Design review of the part built by this model. Coordinates are the model's own, in mm. A direction names the side the tool comes from. Coordinates: 2 decimals unless noted, no trailing zeros. Write each loop counter-clockwise with the first axis right and the second up, starting at its lowest first coordinate (ties: lowest second). Pieces come first, ordered by that corner, then holes. Notation, with made-up numbers: (-7, 17.5) -> (35, 17.5) arc R21 cw to (35, 28.5) -> close; hole circle Ø11 at (53.5, 52). An arc over 180 degrees is marked (long way). Return JSON: item names as keys, results as strings. Group by question number.
from build123d import *

# Parameters (mm, degrees)
BOSS_EXTRUDE1_DEPTH = 9
CUT_EXTRUDE1_DEPTH  = 52
SKETCH4_W           = 7.545775994
SKETCH4_H           = 9.202794467
SKETCH4_W_2         = 8.134906164
CUT_EXTRUDE2_DEPTH  = 25


with BuildPart() as part:
    # Sketch2 → Boss-Extrude1 (new body)
    with BuildSketch(Plane.XY):
        with BuildLine():
            Line((-10.152941176, 19.036764706), (-10.152941176, 26.411764706))
            Line((-10.152941176, 26.411764706), (-38.352941176, 26.411764706))
            Line((-38.352941176, 26.411764706), (-38.352941176, -24.588235294))
            Line((-38.352941176, -24.588235294), (27.647058824, -24.588235294))
            Line((27.647058824, -24.588235294), (27.647058824, 26.411764706))
            Line((27.647058824, 26.411764706), (-0.552941176, 26.411764706))
            Line((-0.552941176, 26.411764706), (-0.552941176, 19.036764706))
            ThreePointArc((-0.552941176, 19.036764706), (-5.352941176, 14.236764706), (-10.152941176, 19.036764706))
        make_face()
    extrude(amount=BOSS_EXTRUDE1_DEPTH)

    # Sketch3 → Cut-Extrude1 (cut, through all)
    with BuildSketch(Plane(origin=(0, 26.411764706, 0), x_dir=(1, 0, 0), z_dir=(0, 1, 0))):
        Polygon((28.053319282, 0), (20.402615126, -2.05), (20.402615126, 0), align=None)
        Polygon((28.053319282, -9), (20.402615126, -6.95), (20.402615126, -9), align=None)
        Polygon((-38.759201635, 0), (-31.108497479, -2.05), (-31.108497479, 0), align=None)
        Polygon((-38.759201635, -9), (-31.108497479, -6.95), (-31.108497479, -9), align=None)
    extrude(amount=-CUT_EXTRUDE1_DEPTH, mode=Mode.SUBTRACT)

    # Sketch4 → Cut-Extrude2 (cut)
    with BuildSketch(Plane.XZ.offset(24.588235294)):
        with Locations((-34.881385476, 4.601397234)):
            Rectangle(SKETCH4_W, SKETCH4_H)
        with Locations((24.470068208, 4.601397234)):
            Rectangle(SKETCH4_W_2, SKETCH4_H)
    extrude(amount=-CUT_EXTRUDE2_DEPTH, mode=Mode.SUBTRACT)


solid = part.part
Q1. We need section A-A on y = 20.5. Write out the cut boundary in (x, z), plus the area to 3 significant figures.
Q2. We need section D-D on y = 3.5. Write out the cut boundary in (x, z).
Q3. For faces 5 (the flat face through (-34.781, 13.594, 7.934)), 6 (the flat face through (-34.781, 13.594, 1.066)), 7 (the flat face through (20.403, -4, 5)), list the 3-axis set-ups (+Z, -Z, +X, -X, +Y, -Y) from which the entire face can be reached by the end or side of a thin tool; tool diameter is ignored.
Q4. We need section C-C on z = 4.25. Write out the cut boundary in (x, y).
Q5. The part is to be moulded in two halves that separate along X. For faces 1 (the flat face through (14, 26.412, 4)), 2 (the flat face through (27.647, 13, 4)), 3 (the flat face through (-31.108, -4, 5)), 4 (the flat face through (-38.353, 14, 4)), say which applies: +X half, -X half, draft (parallel to the pull), parting line (faces both ways), or undercut.
Q6. We need section B-B on z = 1. Write out the cut boundary in (x, y).
Q7. For P1, Ø3.5, axis at x = 23, z = 5, coming from the -Y side; P2, Ø2.5, axis at y = -10, z = 4.5, coming from the -X side; P3, Ø1.5, axis at y = -14.5, z = 3, coming from the +X side, all flat-tipped, find the tip position at first contact; note any pin that passes through.
Q8. Wall thickness on L1, parallel to X at y = 20, z = 6.5; L2, parallel to X at y = -10.5, z = 4; L3, parallel to Y at x = 21, z = 6: over which ranges is each line inside the solid? List them lowest first.
Findings below:
{
 "1": {"outline": "(-38.35, 0.11) -> (-31.11, 2.05) -> (-31.11, 0) -> (-10.15, 0) -> (-10.15, 9) -> (-31.11, 9) -> (-31.11, 6.95) -> (-38.35, 8.89) -> close; (-0.55, 0) -> (20.4, 0) -> (20.4, 2.05) -> (27.65, 0.11) -> (27.65, 8.89) -> (20.4, 6.95) -> (20.4, 9) -> (-0.55, 9) -> close", "area": "476 mm^2"},
 "2": {"outline": "(-38.35, 0.11) -> (-31.11, 2.05) -> (-31.11, 0) -> (20.4, 0) -> (20.4, 2.05) -> (27.65, 0.11) -> (27.65, 8.89) -> (20.4, 6.95) -> (20.4, 9) -> (-31.11, 9) -> (-31.11, 6.95) -> (-38.35, 8.89) -> close"},
 "3": {"face 5": "+Z, +Y, -Y", "face 6": "-Z, +Y, -Y", "face 7": "-Y"},
 "4": {"outline": "(-38.35, 0.41) -> (-31.11, 0.41) -> (-31.11, -24.59) -> (20.4, -24.59) -> (20.4, 0.41) -> (27.65, 0.41) -> (27.65, 26.41) -> (-0.55, 26.41) -> (-0.55, 19.04) arc R4.8 cw to (-10.15, 19.04) -> (-10.15, 26.41) -> (-38.35, 26.41) -> close"},
 "5": {"face 1": "draft", "face 2": "+X half", "face 3": "undercut", "face 4": "-X half"},
 "6": {"outline": "(-38.35, 0.41) -> (-35.03, 0.41) -> (-35.03, 26.41) -> (-38.35, 26.41) -> close; (-31.11, -24.59) -> (20.4, -24.59) -> (20.4, 26.41) -> (-0.55, 26.41) -> (-0.55, 19.04) arc R4.8 cw to (-10.15, 19.04) -> (-10.15, 26.41) -> (-31.11, 26.41) -> close; (24.32, 0.41) -> (27.65, 0.41) -> (27.65, 26.41) -> (24.32, 26.41) -> close"},
 "7": {"P1": "stops at y = 0.41", "P2": "stops at x = -31.11", "P3": "stops at x = 20.4"},
 "8": {"L1": "x = -38.35 to -10.15, -0.55 to 27.65", "L2": "x = -31.11 to 20.4", "L3": "y = 0.41 to 26.41"}
}
